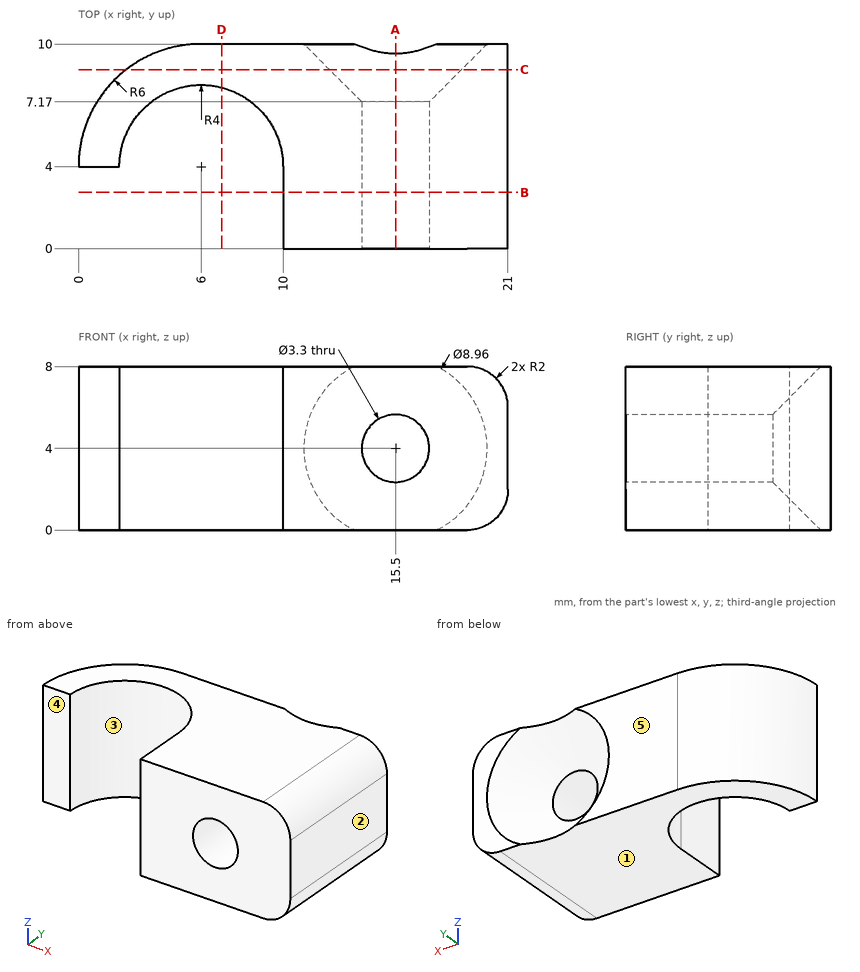
Study the drawing (mm; zero at the part's minimum x, y, z) and answer. A direction names the side the tool comes from. Give positions to 0.01 mm unless a question says otherwise; leave off trailing zeros. Write each loop counter-clockwise with the first axis right and the second up, starting at its lowest first coordinate (ties: lowest second). Pieces come first, ordered by that corner, then holes. Notation, with made-up numbers: M 44,27.5 L 100,27.5 A8 ccw 100,35.5 Z; hole C 6.5,37 d10. An arc over 180 degrees is marked long. Put each result on its own line as item: value. Start each with the question number.
1. Each of these flat-tipped pins is pushed along its axis until it touches: pin 1 Ø4 at (x, z) = (15.5, 4) entering from +Y; pin 2 Ø3 at (y, z) = (1, 3.5) entering from -X; pin 3 Ø0.6 at (x, z) = (0.5, 2) entering from -Y. Where does it stop, or does it pass through?
2. The part is cut by section C-C, the plane y = 8.75. Give the vertices of the cut face in (x, z).
3. Consider line 1 along X through (y, z) = (6.25, 3.25); line 2 along X through (y, z) = (6, 2.75); line 3 along Z through (x, y) = (15.5, 2). Determine where each line is inside the solid, lowest interval first.
4. The part is cut by section D-D, the plane x = 7. Give the vertices of the cut face in (y, z).
5. The part is cut by section B-B, the plane y = 2.75. Give the vertices of the cut face in (x, z), and give its area (3 significant figures).
6. The part is cut by section A-A, the plane x = 15.5. Give the vertices of the cut face in (y, z), and give its area (3 significant figures).
7. Which of the six approach directions +Z, -Z, +X, -X, +Y, -Y give full straight-line access (tool end or side, diameter ignored) to the marked faces 4 and 5?
8. For a pull along X with two mould halves and no side action, classify the marked faces 1, 2 and 3 as released by +X, released by -X, zero draft, split by the parting line, or undercut.
Final values:
1. pin 1: stops at y = 7.52
1. pin 2: stops at x = 10
1. pin 3: stops at y = 4
2. outline: M 2.33,0 L 19,0 A2 ccw 21,2 L 21,6 A2 ccw 19,8 L 2.33,8 Z; hole C 15.5,4 d6.46
3. line 1: x = 0.44 to 2.69, 9.31 to 14.03, 16.97 to 21
3. line 2: x = 0.34 to 2.54, 9.46 to 14.42, 16.58 to 21
3. line 3: z = 0 to 2.35, 5.65 to 8
4. outline: M 7.87,0 L 10,0 L 10,8 L 7.87,8 Z
5. outline: M 10,0 L 19,0 A2 ccw 21,2 L 21,6 A2 ccw 19,8 L 10,8 Z; hole C 15.5,4 d3.3
5. area: 77.7 mm²
6. outline: M 0,0 L 9.52,0 L 7.17,2.35 L 0,2.35 Z; M 0,5.65 L 7.17,5.65 L 9.52,8 L 0,8 Z
6. area: 39.2 mm²
7. face 4: +Z, -Z, -X, -Y
7. face 5: +Z, -Z, +X, -X, +Y
8. face 1: zero draft
8. face 2: released by +X
8. face 3: undercut
